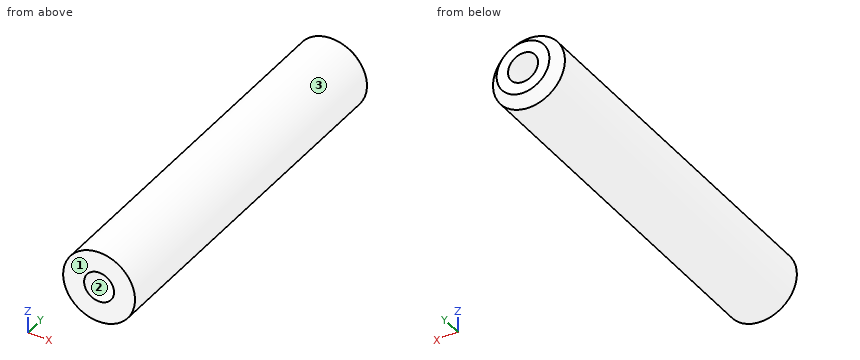
Autodesk Inventor part; units mm, degrees
ref_plane "YZ Plane" through (0, 0, 0) normal (1, 0, 0) x (0, 1, 0)
ref_plane "XZ Plane" through (0, 0, 0) normal (0, 1, 0) x (-1, 0, 0)
ref_plane "XY Plane" through (0, 0, 0) normal (0, 0, 1) x (1, 0, 0)
sketch "Skizze1" plane through (0, 0, 0) normal (0, 1, 0) x (-1, 0, 0)
  circle A0 centre (0, 0) radius 15
  dimension "d0" = 30
extrude "Extrusion1" add sketch "Skizze1" along normal blind 160
chamfer "Fasen1" distance 4 angle 45 1 edges at (15, 160, 0)
sketch "Skizze2" plane through (0, 0, 0) normal (0, -1, 0) x (1, 0, 0)
  circle A0 centre (0, 0) radius 11
  circle A1 centre (0, 0) radius 6.25
  dimension "d6" = 12.5
extrude "Extrusion2" cut sketch "Skizze2" against normal up to surface (160 mm away) contours A1
properties part number "15" material "Kupfer, Guss"
Model file for the job. Use its own axes, mm. Face numbers are marked on the shaded views. Give positions to 0.01 mm unless a question says otherwise; leave off trailing zeros. Write each loop counter-clockwise with the first axis right and the second up, starting at its lowest first coordinate (ties: lowest second). Pieces come first, ordered by that corner, then holes. Notation, with made-up numbers: M 58.5,49.5 L 87.5,49.5 A17 cw 87.5,70.5 Z; hole C 53,-4 d11. An arc over 180 degrees is marked long. One line per item, written item: value. Start each with the question number.
Q1. Two-plate mould, pull along Z, no slides. Class the marked faces 1, 2 and 3: +Z half, -Z half, draft (parallel to the pull), parting line (faces both ways), or undercut.
Q2. Drop flat-ended pins along their axis: pin 1 Ø4 at (x, y) = (7.5, 50.5) entering from -Z; pin 2 Ø3 at (x, y) = (-8.5, 46) entering from +Z; pin 3 Ø1 at (x, y) = (6.5, 36) entering from +Z. Give the stop position or say it passes through.
Q3. Probe probe 1 along Z at (x, y) = (0, 100); probe 2 along X at (y, z) = (24, 0.5); probe 3 along X at (y, z) = (61, -4.5). List the from-to ranges inside material, lowest first. Write a range as [from, to].
Q4. Saw through at A-A, the plane z = 0. Write the cut outline in (x, y), plus the area to 3 significant figures.
Q5. Saw through at B-B, the plane x = 0. Write the cut outline in (y, z).
Q6. Saw through at C-C, the plane y = 36. Write the cut outline in (x, z).
Output values:
1. face 1: draft
1. face 2: undercut
1. face 3: parting line
2. pin 1: stops at z = -13.96
2. pin 2: stops at z = 13.27
2. pin 3: stops at z = 13.75
3. probe 1: z = [-15, -6.25], [6.25, 15]
3. probe 2: x = [-14.99, -6.23], [6.23, 14.99]
3. probe 3: x = [-14.31, -4.34], [4.34, 14.31]
4. outline: M -15,0 L -6.25,0 L -6.25,160 L -11,160 L -15,156 Z; M 6.25,0 L 15,0 L 15,156 L 11,160 L 6.25,160 Z
4. area: 2,780 mm²
5. outline: M 0,-15 L 156,-15 L 160,-11 L 160,-6.25 L 0,-6.25 Z; M 0,6.25 L 160,6.25 L 160,11 L 156,15 L 0,15 Z
6. outline: C 0,0 d30; hole C 0,0 d12.5
